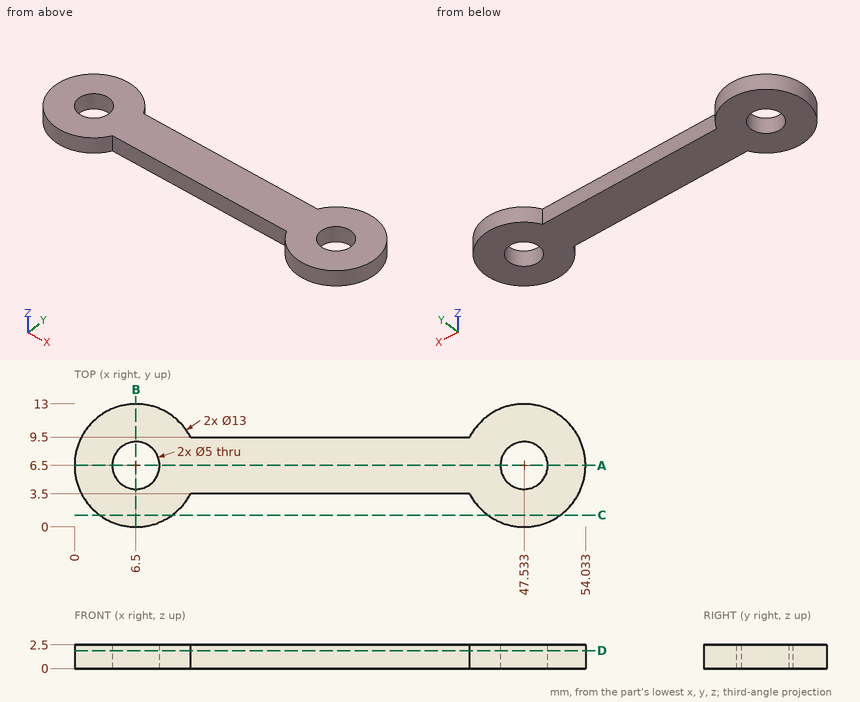
Could you check a few things on this drawing? It's one solid part, dimensions in mm from its lowest x, y, z. Coordinates: 2 decimals unless noted, no trailing zeros. Loops run counter-clockwise (first coordinate to the right, second up) from the corner with the lowest first, then second, coordinate; pieces in that order, holes last.
1. Imagine slicing it at A-A (y = 6.5). Please give me the cut outline in (x, z).
2. Imagine slicing it at C-C (y = 1.25). Please give me the cut outline in (x, z) (1 decimal).
3. Imagine slicing it at D-D (z = 1.9). Please give me the cut outline in (x, y).
4. Imagine slicing it at B-B (x = 6.5). Please give me the cut outline in (y, z), and give its area (3 significant figures).
5. For P1, Ø1.5, axis at y = 9, z = 1, coming from the -X side; P2, Ø3, axis at x = 6.5, y = 6.5, coming from the -Z side, each with a flat end and sliding along its axis, tell me the tip position at first contact or that it passes through.
6. I need wall thicknesses on L1, parallel to X at y = 6.5, z = 0.85; L2, parallel to X at y = 8.5, z = 2.3 (1 decimal); L3, parallel to X at y = 2.5, z = 0.9 (1 decimal). Which ranges of each line are inside material? Lowest first, please.
Computed values:
1. outline: (0, 0) - (4, 0) - (4, 2.5) - (0, 2.5) - close; (9, 0) - (45.03, 0) - (45.03, 2.5) - (9, 2.5) - close; (50.03, 0) - (54.03, 0) - (54.03, 2.5) - (50.03, 2.5) - close
2. outline: (2.7, 0) - (10.3, 0) - (10.3, 2.5) - (2.7, 2.5) - close; (43.7, 0) - (51.4, 0) - (51.4, 2.5) - (43.7, 2.5) - close
3. outline: (12.27, 3.5) - (41.77, 3.5) arc R6.5 ccw (long way) to (41.77, 9.5) - (12.27, 9.5) arc R6.5 ccw (long way) to start; hole circle Ø5 at (6.5, 6.5); hole circle Ø5 at (47.53, 6.5)
4. outline: (0, 0) - (4, 0) - (4, 2.5) - (0, 2.5) - close; (9, 0) - (13, 0) - (13, 2.5) - (9, 2.5) - close
4. area: 20.0 mm2
5. P1: stops at x = 0.24
5. P2: passes through
6. L1: x = 0 to 4, 9 to 45.03, 50.03 to 54.03
6. L2: x = 0.3 to 5, 8 to 46, 49 to 53.7
6. L3: x = 1.4 to 11.6, 42.4 to 52.7
